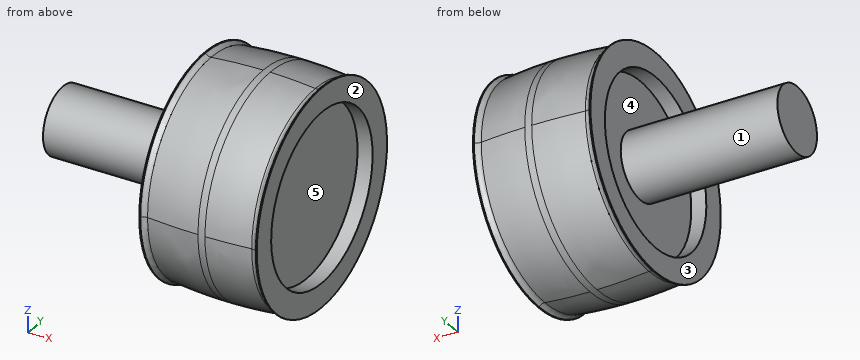
```python
from build123d import *

# Parameters (mm, degrees)
BOSS_EXTRU_1_DEPTH      = 9.75
BOSS_EXTRU_1_DEPTH_BACK = 9.75
ESQUISSE2_R             = 18.08
ESQUISSE4_R             = 14.08
ENL_V_MAT_EXTRU_1_DEPTH = 2.5
ENL_V_START             = -2.5
ESQUISSE5_R             = 14.08
ENL_V_MAT_EXTRU_2_DEPTH = 2.5
ESQUISSE6_R             = 5.5
BOSS_EXTRU_2_DEPTH      = 26


with BuildPart() as part:
    # Esquisse2 → Boss.-Extru.1 (new, two sides: drawn at the far end of the back side and taken through both)
    with BuildSketch(Plane(origin=(0, 0, 0), x_dir=(0, 0, -1), z_dir=(1, 0, 0)).offset(-BOSS_EXTRU_1_DEPTH_BACK)):
        with Locations((0, -30.697276077)):
            Circle(ESQUISSE2_R)
    extrude(amount=BOSS_EXTRU_1_DEPTH + BOSS_EXTRU_1_DEPTH_BACK)

    # Enl_vement de mati_re-Balayage1: sweep along a curve in space
    with BuildLine() as enl_vement_de_mati_re_balayage1_path:
        ThreePointArc((9.75, -30.697276077, -18.08), (9.75, -17.912785473, -12.784490604), (9.75, -12.617276077, 0))
        ThreePointArc((9.75, -12.617276077, 0), (9.75, -17.912785473, 12.784490604), (9.75, -30.697276077, 18.08))
        ThreePointArc((9.75, -30.697276077, 18.08), (9.75, -43.481766681, 12.784490604), (9.75, -48.777276077, 0))
        ThreePointArc((9.75, -48.777276077, 0), (9.75, -43.481766681, -12.784490604), (9.75, -30.697276077, -18.08))
    # Esquisse1 → Enl_vement de mati_re-Balayage1 (sweep, cut)
    with BuildSketch(Plane.XY):
        with BuildLine():
            Line((9.75, -1.705844805), (9.75, -12.080482835))
            ThreePointArc((9.75, -12.080482835), (9.418659658, -12.824051434), (8.644211477, -13.074871486))
            add(Edge.make_bspline(
                [(-8.639497918, -13.06789707), (-5.962658662, -12.770278108), (1.018950966, -12.480757929), (5.401157061, -12.729857554), (8.644211477, -13.074871486)],
                knots=[0.057340546, 0.057340546, 0.057340546, 0.057340546, 0.473274059, 0.946548119, 0.946548119, 0.946548119, 0.946548119], degree=3))
            ThreePointArc((-8.639497918, -13.06789707), (-9.416895013, -12.819172867), (-9.75, -12.074021177))
            Line((-9.75, -12.074021177), (-9.75, -1.69364433))
            ThreePointArc((-9.75, -1.69364433), (-9.265544866, -0.388606491), (-8.04687624, 0.284199066))
            add(Edge.make_bspline(
                [(-8.04687624, 0.284199066), (-5.709420251, 0.63505351), (1.539056453, 0.939568483), (5.000411491, 0.71370426), (8.036962294, 0.273461297)],
                knots=[0.08950135, 0.08950135, 0.08950135, 0.08950135, 0.457115955, 0.91423191, 0.91423191, 0.91423191, 0.91423191], degree=3))
            ThreePointArc((8.036962294, 0.273461297), (9.262270576, -0.397014141), (9.75, -1.705844805))
        make_face()
    sweep(path=enl_vement_de_mati_re_balayage1_path.line, mode=Mode.SUBTRACT)

    # Esquisse4 → Enl_v. mat.-Extru.1 (cut)
    with BuildSketch(Plane(origin=(9.75, 0, 0), x_dir=(0, 0, -1), z_dir=(1, 0, 0))):
        with Locations((0, -30.697276077)):
            Circle(ESQUISSE4_R)
    extrude(amount=-ENL_V_MAT_EXTRU_1_DEPTH, mode=Mode.SUBTRACT)

    # Esquisse5 → Enl_v. mat.-Extru.2 (cut)
    with BuildSketch(Plane.ZY.offset(9.75).offset(ENL_V_START)):
        with Locations(Location((0, -30.697276077, 0), (0, 0, 180))):
            Circle(ESQUISSE5_R)
    extrude(amount=ENL_V_MAT_EXTRU_2_DEPTH, mode=Mode.SUBTRACT)

    # Esquisse6 → Boss.-Extru.2 (add)
    with BuildSketch(Plane.ZY.offset(7.25)):
        with Locations(Location((0, -30.697276077, 0), (0, 0, 180))):
            Circle(ESQUISSE6_R)
    extrude(amount=BOSS_EXTRU_2_DEPTH)


solid = part.part
```
Source: CAD feature listing. Evaluate the final solid. Frame: model axes, mm. Face numbers are marked on the shaded views. A direction names the side the tool comes from. Round coordinates to 2 decimals unless told otherwise and drop trailing zeros. Order: outer loops, then holes, each group sorted by start corner. A loop starts at its lowest first (then second) coordinate and runs counter-clockwise, first axis right, second up. Notation, with made-up numbers: (-24.5, 49) -> (16.5, 49) arc R5 cw to (16.5, 55) -> close; hole circle Ø2 at (60.5, -29.5). An arc over 180 degrees is marked (long way). One line per item, written item: value. Start each with the question number.
Q1. Section query A-A (x = -26). Return the cut outline in (y, z).
Q2. Pin query (flat end, axial travel): pin 1 (1.5 mm diameter, centred on y = -19.5, z = -3.5, fed in from +X); pin 2 (8 mm diameter, centred on x = -20, z = 13, fed in from +Y); pin 3 (6 mm diameter, centred on x = -10.5, z = -14, fed in from -Y); pin 4 (4 mm diameter, centred on y = -21.5, z = 11, fed in from -X). Return the tip coordinate at first contact, or that it passes through.
Q3. Material intervals for probe 1 along X at (y, z) = (-20.5, -9.5); probe 2 along X at (y, z) = (-44, -10.5); probe 3 along Z at (x, y) = (-8, -27), sorted ascending.
Q4. Access query for the marked faces 1 and 2. Directions: +Z, -Z, +X, -X, +Y, -Y. A direction counts if a zero-diameter tool reaches every point of the face in a straight line with its end or side. Return the directions, or none.
Q5. Draft query along Z for the marked faces 3, 4 and 5. Return one class per face: pulls with the +Z half, pulls with the -Z half, needs draft (parallel to the pull), parting line crosses it, or undercut.
Findings below:
1. outline: circle Ø11 at (-30.7, 0)
2. pin 1: x = 7.25
2. pin 2: through
2. pin 3: y = -44.97
2. pin 4: x = -9.75
3. probe 1: -7.25 to 7.25
3. probe 2: -9.75 to 9.75
3. probe 3: -17.31 to -13.59, -4.07 to 4.07, 13.59 to 17.31
4. face 1: -X
4. face 2: +Z, -Z, +X, +Y, -Y
5. face 3: needs draft
5. face 4: undercut
5. face 5: undercut
